Model file for the job. Use its own axes, mm. A direction names the side the tool comes from. Give positions to 0.01 mm unless a question says otherwise; leave off trailing zeros. Write each loop counter-clockwise with the first axis right and the second up, starting at its lowest first coordinate (ties: lowest second). Pieces come first, ordered by that corner, then holes. Notation, with made-up numbers: (19.25, 3) - (23.25, 3) arc R19 cw to (23.25, 38) - close; hole circle Ø3 at (31, 83). An arc over 180 degrees is marked (long way). One line per item, written item: value. Start each with the question number.
(1) Cut at B-B, the plane y = -16. List the corners of the cut face in (x, z).
(2) Cut at C-C, the plane x = -15. List the corners of the cut face in (y, z).
(3) Probe L1, parallel to Y at x = 76.5, z = 427; L2, parallel to Z at x = 43, y = 21.5; L3, parallel to X at y = 90, z = 424.5. List the from-to ranges inside material, lowest first.
(4) Cut at A-A, the plane z = 440.5. List the corners of the cut face in (x, y), and give its area (3 significant figures).
(5) 3-axis set-ups, long thin cutter, end or side, ignore diameter. For faces 4 (the face through (-1, 37.5, 435)), 5 (the face through (-100, -1.1, 414.8)): which of +Z, -Z, +X, -X, +Y, -Y reach the whole face in a straight line?
(6) Mould opens along Y. For faces 1 (the face through (94.297, 1.12, 376.014)), 2 (the face through (-1, -37.5, 435)), 3 (the face through (-1, -100, 422)) say: pulls with the +Y half, pulls with the -Y half, needs draft (parallel to the pull), parting line crosses it, or undercut.
(7) Drop flat-ended pins along their axis: P1, Ø8, axis at x = -25.5, y = 23, coming from the +Z side; P2, Ø2, axis at y = 75, z = 387.5, coming from the -X side. Give the stop position or say it passes through.
from build123d import *

# Parameters (mm, degrees)
SKETCH003_W  = 200
SKETCH003_H  = 200
PAD003_DEPTH = 45
SKETCH009_W  = 200
SKETCH009_H  = 62.5
PAD009_DEPTH = 40
FILLET005_R  = 20


with BuildPart() as part:
    # Sketch003 (on Face1 of CopyPad002) → Pad003 (new body)
    with BuildSketch(Plane.XY.offset(370)):
        Rectangle(SKETCH003_W, SKETCH003_H)
    extrude(amount=PAD003_DEPTH)

    # Sketch009 (on Face6 of Pad003) → Pad009 (join)
    with BuildSketch(Plane.XY.offset(415)):
        with Locations((0, 68.75)):
            Rectangle(SKETCH009_W, SKETCH009_H)
        with Locations((0, -68.75)):
            Rectangle(SKETCH009_W, SKETCH009_H)
    extrude(amount=PAD009_DEPTH)

    # Fillet005
    fillet005_edges = [part.edges().sort_by_distance(p)[0] for p in [
        (-100, -100, 412.5),
        (100, -100, 412.5),
        (100, 100, 412.5),
        (-100, 100, 412.5),
        (0, -100, 370),
        (100, 0, 370),
        (-100, 0, 370),
        (0, 100, 370),
    ]]
    fillet(fillet005_edges, radius=FILLET005_R)


solid = part.part
Answers follow:
1. outline: (-100, 390) arc R20 ccw to (-80, 370) - (80, 370) arc R20 ccw to (100, 390) - (100, 415) - (-100, 415) - close
2. outline: (-100, 390) arc R20 ccw to (-80, 370) - (80, 370) arc R20 ccw to (100, 390) - (100, 455) - (37.5, 455) - (37.5, 415) - (-37.5, 415) - (-37.5, 455) - (-100, 455) - close
3. L1: y = -100 to -37.5, 37.5 to 100
3. L2: z = 370 to 415
3. L3: x = -97.32 to 97.32
4. outline: (-100, -80) arc R20 ccw to (-80, -100) - (80, -100) arc R20 ccw to (100, -80) - (100, -37.5) - (-100, -37.5) - close; (-100, 37.5) - (100, 37.5) - (100, 80) arc R20 ccw to (80, 100) - (-80, 100) arc R20 ccw to (-100, 80) - close
4. area: 24,700 mm²
5. face 4: +Z, +X, -X
5. face 5: +Z, -Z, -X, +Y, -Y
6. face 1: needs draft
6. face 2: undercut
6. face 3: pulls with the -Y half
7. P1: stops at z = 415
7. P2: stops at x = -99.94
